Part model, mm, in its own coordinate system. A direction names the side the tool comes from. Give positions to 0.01 mm unless a question says otherwise; leave off trailing zeros. Order: outer loops, then holes, each group sorted by start corner. A loop starts at its lowest first (then second) coordinate and runs counter-clockwise, first axis right, second up. Notation, with made-up numbers: M -10,-14 L 39,-14 A11 ccw 39,5 Z; hole C 23.25,26 d3. An arc over 180 degrees is marked long. One line per question, with ' | ' between items.
```python
from build123d import *

# Parameters (mm, degrees)
SKETCH1_W            = 75
SKETCH1_H            = 75
MAINSHAPE_DEPTH      = 4.5
SKETCH5_W            = 4.35
SKETCH5_H            = 9.7
CUT_EXTRUDE3_DEPTH   = 54.223584998
CUT_EXTRUDE4_DEPTH   = 54.223584998
BOSS_EXTRUDE2_DEPTH  = 4.5
SKETCH8_R            = 1.45
CUT_EXTRUDE6_DEPTH   = 60.51890456
SKETCH11_W           = 10
SKETCH11_H           = 4.5
REARTABS_DEPTH       = 4.5
FRONTSCREWSLOT_DEPTH = 63.451981554
SKETCH14_R           = 1.45
BRACESCREWS_DEPTH    = 63.451981554
WIRINGSLOT_DEPTH     = 63.451981554
BOSS_EXTRUDE4_DEPTH  = 4.5


with BuildPart() as part:
    # Sketch1 → MainShape (new body)
    with BuildSketch(Plane(origin=(0, 0, 0), x_dir=(1, 0, 0), z_dir=(0, 1, 0))):
        Rectangle(SKETCH1_W, SKETCH1_H)
    extrude(amount=MAINSHAPE_DEPTH)

    # Sketch5 → Cut-Extrude3 (cut, through all)
    with BuildSketch(Plane(origin=(0, 4.5, 0), x_dir=(1, 0, 0), z_dir=(0, 1, 0))):
        with Locations((33, 22.5)):
            Rectangle(SKETCH5_W, SKETCH5_H)
        with Locations((-33, 22.5)):
            Rectangle(SKETCH5_W, SKETCH5_H)
        with Locations((-33, -17.5)):
            Rectangle(SKETCH5_W, SKETCH5_H)
        with Locations((33, -17.5)):
            Rectangle(SKETCH5_W, SKETCH5_H)
    extrude(amount=-CUT_EXTRUDE3_DEPTH, mode=Mode.SUBTRACT)

    # Sketch6 → Cut-Extrude4 (cut, through all)
    with BuildSketch(Plane(origin=(0, 4.5, 0), x_dir=(1, 0, 0), z_dir=(0, 1, 0))):
        with BuildLine():
            Line((-24, -15.5), (-24, -7.520797289))
            ThreePointArc((-24, -7.520797289), (-18, 7), (-12, -7.520797289))
            Line((-12, -7.520797289), (-12, -15.5))
            ThreePointArc((-12, -15.5), (-18, -21.5), (-24, -15.5))
        make_face()
    cut_extrude4 = extrude(amount=-CUT_EXTRUDE4_DEPTH, mode=Mode.SUBTRACT)

    # Sketch13 → Boss-Extrude2 (add, through all)
    with BuildSketch(Plane(origin=(0, 4.5, 0), x_dir=(1, 0, 0), z_dir=(0, 1, 0))):
        Polygon((-37.5, -37.5), (-37.5, 0), (-46, -7.5), (-46, -37.5), align=None)
        Polygon((37.5, 0), (37.5, -37.5), (46, -37.5), (46, -7.5), align=None)
    extrude(amount=-BOSS_EXTRUDE2_DEPTH)

    # Sketch8 → Cut-Extrude6 (cut, through all)
    with BuildSketch(Plane(origin=(0, 4.5, 0), x_dir=(1, 0, 0), z_dir=(0, 1, 0))):
        with Locations(Location((-39.46, -7.5, 0), (0, 0, 270))):
            Circle(SKETCH8_R)
        with Locations(Location((-39.46, -23.5, 0), (0, 0, 270))):
            Circle(SKETCH8_R)
    cut_extrude6 = extrude(amount=-CUT_EXTRUDE6_DEPTH, mode=Mode.SUBTRACT)

    # Mirror1: Cut-Extrude4, Cut-Extrude6 across plane
    add(cut_extrude4.mirror(Plane(origin=(0, 0, 0), x_dir=(0, 0, 1), z_dir=(1, 0, 0))), mode=Mode.SUBTRACT)
    add(cut_extrude6.mirror(Plane(origin=(0, 0, 0), x_dir=(0, 0, 1), z_dir=(1, 0, 0))), mode=Mode.SUBTRACT)

    # Sketch11 → RearTabs (add, through all)
    with BuildSketch(Plane(origin=(0, 4.5, 0), x_dir=(1, 0, 0), z_dir=(0, 1, 0))):
        with Locations((-25, 39.75)):
            Rectangle(SKETCH11_W, SKETCH11_H)
        with Locations((25, 39.75)):
            Rectangle(SKETCH11_W, SKETCH11_H)
    extrude(amount=-REARTABS_DEPTH)

    # Sketch12 → FrontScrewSlot (cut, through all)
    with BuildSketch(Plane(origin=(0, 4.5, 0), x_dir=(1, 0, 0), z_dir=(0, 1, 0))):
        with BuildLine():
            Line((-13.45, 37.5), (-16.55, 37.5))
            Line((-16.55, 37.5), (-16.55, 33))
            Line((-16.55, 33), (-17.35, 33))
            ThreePointArc((-17.35, 33), (-17.703553391, 32.853553391), (-17.85, 32.5))
            Line((-17.85, 32.5), (-17.85, 30))
            ThreePointArc((-17.85, 30), (-17.703553391, 29.646446609), (-17.35, 29.5))
            Line((-17.35, 29.5), (-16.55, 29.5))
            Line((-16.55, 29.5), (-16.55, 25.5))
            Line((-16.55, 25.5), (-13.45, 25.5))
            Line((-13.45, 25.5), (-13.45, 29.5))
            Line((-13.45, 29.5), (-12.65, 29.5))
            ThreePointArc((-12.65, 29.5), (-12.296446609, 29.646446609), (-12.15, 30))
            Line((-12.15, 30), (-12.15, 32.5))
            ThreePointArc((-12.15, 32.5), (-12.296446609, 32.853553391), (-12.65, 33))
            Line((-12.65, 33), (-13.45, 33))
            Line((-13.45, 33), (-13.45, 37.5))
        make_face()
        with BuildLine():
            Line((13.45, 37.5), (13.45, 33))
            Line((13.45, 33), (12.65, 33))
            ThreePointArc((12.65, 33), (12.296446609, 32.853553391), (12.15, 32.5))
            Line((12.15, 32.5), (12.15, 30))
            ThreePointArc((12.15, 30), (12.296446609, 29.646446609), (12.65, 29.5))
            Line((12.65, 29.5), (13.45, 29.5))
            Line((13.45, 29.5), (13.45, 25.5))
            Line((13.45, 25.5), (16.55, 25.5))
            Line((16.55, 25.5), (16.55, 29.5))
            Line((16.55, 29.5), (17.35, 29.5))
            ThreePointArc((17.35, 29.5), (17.703553391, 29.646446609), (17.85, 30))
            Line((17.85, 30), (17.85, 32.5))
            ThreePointArc((17.85, 32.5), (17.703553391, 32.853553391), (17.35, 33))
            Line((17.35, 33), (16.55, 33))
            Line((16.55, 33), (16.55, 37.5))
            Line((16.55, 37.5), (13.45, 37.5))
        make_face()
    extrude(amount=-FRONTSCREWSLOT_DEPTH, mode=Mode.SUBTRACT)

    # Sketch14 → BraceScrews (cut, through all)
    with BuildSketch(Plane(origin=(0, 4.5, 0), x_dir=(1, 0, 0), z_dir=(0, 1, 0))):
        with Locations(Location((-33, -31.5, 0), (0, 0, 270))):
            Circle(SKETCH14_R)
        with Locations(Location((33, -31.5, 0), (0, 0, 270))):
            Circle(SKETCH14_R)
    extrude(amount=-BRACESCREWS_DEPTH, mode=Mode.SUBTRACT)

    # Sketch16 → WiringSlot (cut, through all)
    with BuildSketch(Plane(origin=(0, 4.5, 0), x_dir=(1, 0, 0), z_dir=(0, 1, 0))):
        with BuildLine():
            Line((3, 22.5), (3, 12.5))
            ThreePointArc((3, 12.5), (0, 9.5), (-3, 12.5))
            Line((-3, 12.5), (-3, 22.5))
            ThreePointArc((-3, 22.5), (0, 25.5), (3, 22.5))
        make_face()
    extrude(amount=-WIRINGSLOT_DEPTH, mode=Mode.SUBTRACT)

    # Sketch21 → Boss-Extrude4 (add, through all)
    with BuildSketch(Plane(origin=(0, 4.5, 0), x_dir=(1, 0, 0), z_dir=(0, 1, 0))):
        with BuildLine():
            Line((-37, 37.5), (-43, 37.5))
            ThreePointArc((-43, 37.5), (-45.121320344, 36.621320344), (-46, 34.5))
            Line((-46, 34.5), (-46, 25.5))
            ThreePointArc((-46, 25.5), (-45.121320344, 23.378679656), (-43, 22.5))
            Line((-43, 22.5), (-42, 22.5))
            Line((-42, 22.5), (-42, 29.5))
            ThreePointArc((-42, 29.5), (-41.121320344, 31.621320344), (-39, 32.5))
            Line((-39, 32.5), (-37, 32.5))
            Line((-37, 32.5), (-37, 37.5))
        make_face()
    extrude(amount=-BOSS_EXTRUDE4_DEPTH)


solid = part.part
```
1. Tool access for faces 1 (the flat face through (-13.45, 2, -27)), 2 (the cylindrical face through (-45.1, 2.28, -36.64)), 3 (the flat face through (3, 2, -18)): list every direction of +Z, -Z, +X, -X, +Y, -Y with a clear straight run to the whole face (end or side of a thin tool).
Worked out:
face 1: -Z, +Y, -Y | face 2: -Z, -X, +Y, -Y | face 3: +Y, -Y
2. Slice it at B-B on x = -22. Give the cut face in (y, z).
Worked out:
outline: M 0,-42 L 4.5,-42 L 4.5,-6 L 0,-6 Z; M 0,19.97 L 4.5,19.97 L 4.5,37.5 L 0,37.5 Z
3. Drop flat-ended pins along their axis: pin 1 (2.5 mm diameter, centred on x = 39.46, z = 23.5, fed in from -Y); pin 2 (0.9 mm diameter, centred on x = 15, y = 1.5, fed in from -Z); pin 3 (2 mm diameter, centred on x = 1, y = 4, fed in from -Z); pin 4 (1 mm diameter, centred on y = 1.5, z = -33.5, fed in from +X). Give the stop position or say it passes through.
Worked out:
pin 1: passes through | pin 2: stops at z = -25.5 | pin 3: stops at z = -37.5 | pin 4: stops at x = 37.5
4. Slice it at D-D on y = 2.35. Give the number of separate pieces and of enclosed holes in the cut face, then the cut area to 3 significant figures.
Worked out:
separate pieces: 1 | enclosed holes: 13 | area: 5,260 mm2
5. Slice it at A-A on z = -2.5. Give the cut face in (x, y).
Worked out:
outline: M -37.5,0 L -25.5,0 L -25.5,4.5 L -37.5,4.5 Z; M -10.5,0 L 10.5,0 L 10.5,4.5 L -10.5,4.5 Z; M 25.5,0 L 37.5,0 L 37.5,4.5 L 25.5,4.5 Z
6. Probe L1, parallel to Z at x = -35, y = 4.05; L2, parallel to X at y = 3.35, z = 23.5; L3, parallel to X at y = 2.9, z = 7.5. List the from-to ranges inside material, lowest first. Write a range as from..to.
Worked out:
L1: z = -37.5..-27.35, -17.65..12.65, 22.35..37.5 | L2: x = -46..-40.91, -38.01..38.01, 40.91..46 | L3: x = -46..-40.91, -38.01..-24.02, -11.98..11.98, 24.02..38.01, 40.91..46
7. Mould opens along Z. For faces 4 (the flat face through (-46, 2, 22)), 5 (the flat face through (41.81, 2.282, 3.802)), 6 (the flat face through (-42, 2, -26)), 7 (the flat face through (-41.69, 2.282, 3.698)) say: released by +Z, released by -Z, zero draft, split by the parting line, or undercut.
Worked out:
face 4: zero draft | face 5: released by -Z | face 6: undercut | face 7: undercut
8. Slice it at C-C on x = 39.46. Give the cut face in (y, z).
Worked out:
outline: M 0,1.73 L 4.5,1.73 L 4.5,6.05 L 0,6.05 Z; M 0,8.95 L 4.5,8.95 L 4.5,22.05 L 0,22.05 Z; M 0,24.95 L 4.5,24.95 L 4.5,37.5 L 0,37.5 Z
